Verification items for the finished model (mm, model axes). Give positions to 0.01 mm unless a question says otherwise; leave off trailing zeros. Write each loop counter-clockwise with the first axis right and the second up, starting at its lowest first coordinate (ties: lowest second). Pieces come first, ordered by that corner, then holes. Notation, with made-up numbers: (-18, 9.25) -> (23, 9.25) arc R28 cw to (23, 36.25) -> close; hole circle Ø11 at (-35, 68.25). An arc over 180 degrees is marked (long way). Use CSV: the item, a comma, the result in double quotes. Start each with the question number.
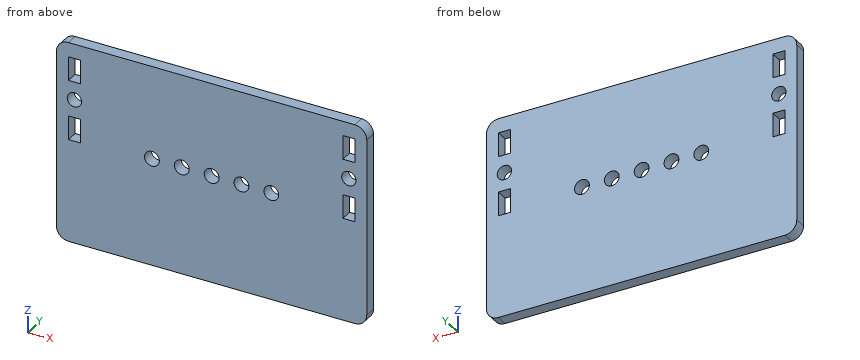
```python
from build123d import *

# Parameters (mm, degrees)
SKETCH1_W           = 130
SKETCH1_H           = 52
BOSS_EXTRUDE1_DEPTH = 5
SKETCH2_W           = 130
SKETCH2_H           = 5
BOSS_EXTRUDE2_DEPTH = 32
SKETCH3_R           = 3
SKETCH3_W           = 5
SKETCH3_H           = 10
CUT_EXTRUDE1_DEPTH  = 10
FILLET1_R           = 5
CUT_EXTRUDE2_REACH  = 89.258
SKETCH4_R           = 3.1


with BuildPart() as part:
    # Sketch1 → Boss-Extrude1 (new body)
    with BuildSketch(Plane(origin=(0, 0, 0), x_dir=(1, 0, 0), z_dir=(0, 1, 0))):
        Rectangle(SKETCH1_W, SKETCH1_H)
    extrude(amount=BOSS_EXTRUDE1_DEPTH)

    # Sketch2 → Boss-Extrude2 (add)
    with BuildSketch(Plane(origin=(0, 0, -26), x_dir=(-1, 0, 0), z_dir=(0, 0, -1))):
        with Locations((0, 2.5)):
            Rectangle(SKETCH2_W, SKETCH2_H)
    extrude(amount=BOSS_EXTRUDE2_DEPTH)

    # Sketch3 → Cut-Extrude1 (cut)
    with BuildSketch(Plane(origin=(0, 5, 0), x_dir=(1, 0, 0), z_dir=(0, 1, 0))):
        with Locations(Location((-57.5, -2.5, 0), (0, 0, 270))):
            Circle(SKETCH3_R)
        with Locations(Location((57.5, -2.5, 0), (0, 0, 270))):
            Circle(SKETCH3_R)
        with Locations((57.5, 10)):
            Rectangle(SKETCH3_W, SKETCH3_H)
        with Locations((-57.5, -15)):
            Rectangle(SKETCH3_W, SKETCH3_H)
        with Locations((-57.5, 10)):
            Rectangle(SKETCH3_W, SKETCH3_H)
        with Locations((57.5, -15)):
            Rectangle(SKETCH3_W, SKETCH3_H)
    extrude(amount=-CUT_EXTRUDE1_DEPTH, mode=Mode.SUBTRACT)

    # Fillet1
    fillet1_edges = [part.edges().sort_by_distance(p)[0] for p in [
        (65, 2.5, -58),
        (-65, 2.5, -58),
        (65, 2.5, 26),
        (-65, 2.5, 26),
    ]]
    fillet(fillet1_edges, radius=FILLET1_R)

    # Sketch4 → Cut-Extrude2 (cut, up to next)
    with BuildSketch(Plane(origin=(0, 5, 0), x_dir=(1, 0, 0), z_dir=(0, 1, 0)), mode=Mode.PRIVATE) as cut_extrude2_sk1:
        with Locations(Location((-12.5, 13, 0), (0, 0, 270))):
            Circle(SKETCH4_R)
    cut_extrude2_tool1 = extrude(cut_extrude2_sk1.sketch, amount=-CUT_EXTRUDE2_REACH, mode=Mode.PRIVATE) & part.part
    # Sketch4 → Cut-Extrude2 (cut, up to next)
    with BuildSketch(Plane(origin=(0, 5, 0), x_dir=(1, 0, 0), z_dir=(0, 1, 0)), mode=Mode.PRIVATE) as cut_extrude2_sk2:
        with Locations(Location((-25, 13, 0), (0, 0, 270))):
            Circle(SKETCH4_R)
    cut_extrude2_tool2 = extrude(cut_extrude2_sk2.sketch, amount=-CUT_EXTRUDE2_REACH, mode=Mode.PRIVATE) & part.part
    # Sketch4 → Cut-Extrude2 (cut, up to next)
    with BuildSketch(Plane(origin=(0, 5, 0), x_dir=(1, 0, 0), z_dir=(0, 1, 0)), mode=Mode.PRIVATE) as cut_extrude2_sk3:
        with Locations(Location((0, 13, 0), (0, 0, 270))):
            Circle(SKETCH4_R)
    cut_extrude2_tool3 = extrude(cut_extrude2_sk3.sketch, amount=-CUT_EXTRUDE2_REACH, mode=Mode.PRIVATE) & part.part
    # Sketch4 → Cut-Extrude2 (cut, up to next)
    with BuildSketch(Plane(origin=(0, 5, 0), x_dir=(1, 0, 0), z_dir=(0, 1, 0)), mode=Mode.PRIVATE) as cut_extrude2_sk4:
        with Locations(Location((12.5, 13, 0), (0, 0, 270))):
            Circle(SKETCH4_R)
    cut_extrude2_tool4 = extrude(cut_extrude2_sk4.sketch, amount=-CUT_EXTRUDE2_REACH, mode=Mode.PRIVATE) & part.part
    # Sketch4 → Cut-Extrude2 (cut, up to next)
    with BuildSketch(Plane(origin=(0, 5, 0), x_dir=(1, 0, 0), z_dir=(0, 1, 0)), mode=Mode.PRIVATE) as cut_extrude2_sk5:
        with Locations(Location((25, 13, 0), (0, 0, 270))):
            Circle(SKETCH4_R)
    cut_extrude2_tool5 = extrude(cut_extrude2_sk5.sketch, amount=-CUT_EXTRUDE2_REACH, mode=Mode.PRIVATE) & part.part
    add(cut_extrude2_tool1.solids().sort_by_distance((-12.5, 5, -13))[0], mode=Mode.SUBTRACT)
    add(cut_extrude2_tool2.solids().sort_by_distance((-25, 5, -13))[0], mode=Mode.SUBTRACT)
    add(cut_extrude2_tool3.solids().sort_by_distance((0, 5, -13))[0], mode=Mode.SUBTRACT)
    add(cut_extrude2_tool4.solids().sort_by_distance((12.5, 5, -13))[0], mode=Mode.SUBTRACT)
    add(cut_extrude2_tool5.solids().sort_by_distance((25, 5, -13))[0], mode=Mode.SUBTRACT)


solid = part.part
```
(1) Section check D-D on x = 0. Record the cut outline in (y, z).
(2) Go/stop test with a flat-tipped pin: pin 1 (5.5 mm diameter, centred on x = 57.5, z = 2.5, fed in from +Y). Record where the tip stops, or that it passes through.
(3) Section check A-A on z = -13. Give the number of separate pieces and of enclosed holes in the cut face, then the cut area to 3 significant figures.
(4) Section check B-B on x = 57.5. Record the cut outline in (y, z), then the cut area to 3 significant figures.
(5) Thickness scan on line 1 (X direction, y = 1.9, z = 2.5); line 2 (X direction, y = 1.2, z = 16.5); line 3 (Z direction, x = -55.5, y = 2.55). Record the ranges inside material, lowest first. Write a range as from..to.
Data:
1,outline,"(0, -58) -> (5, -58) -> (5, -16.1) -> (0, -16.1) -> close; (0, -9.9) -> (5, -9.9) -> (5, 26) -> (0, 26) -> close"
2,pin 1,"passes through"
3,separate pieces,"8"
3,enclosed holes,"0"
3,area,"445 mm2"
4,outline,"(0, -58) -> (5, -58) -> (5, -15) -> (0, -15) -> close; (0, -5) -> (5, -5) -> (5, -0.5) -> (0, -0.5) -> close; (0, 5.5) -> (5, 5.5) -> (5, 10) -> (0, 10) -> close; (0, 20) -> (5, 20) -> (5, 26) -> (0, 26) -> close"
4,area,"290 mm2"
5,line 1,"x = -65..-60.5, -54.5..54.5, 60.5..65"
5,line 2,"x = -65..-60, -55..55, 60..65"
5,line 3,"z = -58..-15, -5..0.26, 4.74..10, 20..26"
